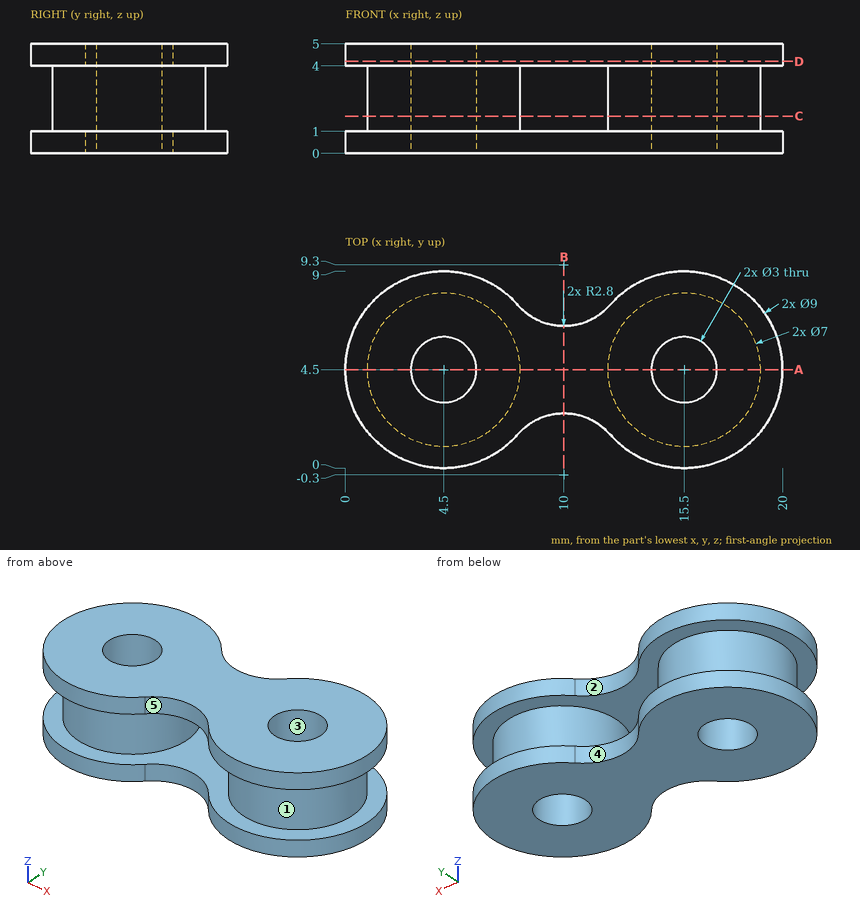
Part print with two shaded views. Sizes in mm from the minimum x, y, z corner. A direction names the side the tool comes from. Give positions to 0.01 mm unless a question says otherwise; leave off trailing zeros. Order: outer loops, then holes, each group sorted by start corner. A loop starts at its lowest first (then second) coordinate and runs counter-clockwise, first axis right, second up. Notation, with made-up numbers: M 55,27.5 L 72,27.5 A19 ccw 72,62.5 Z; hole C 29,87 d2. An arc over 180 degrees is marked long. Use one line per item in the form item = value.
1) Saw through at A-A (y = 4.5). Give the cut face in (x, z), plus the area to 3 significant figures.
Calculated:
outline = M 0,0 L 3,0 L 3,5 L 0,5 L 0,4 L 1,4 L 1,1 L 0,1 Z; M 6,0 L 14,0 L 14,5 L 6,5 Z; M 17,0 L 20,0 L 20,1 L 19,1 L 19,4 L 20,4 L 20,5 L 17,5 Z; hole M 8,1 L 12,1 L 12,4 L 8,4 Z
area = 52.0 mm2
2) Saw through at B-B (x = 10). Give the cut face in (y, z).
Calculated:
outline = M 2.5,0 L 6.5,0 L 6.5,1 L 2.5,1 Z; M 2.5,4 L 6.5,4 L 6.5,5 L 2.5,5 Z
3) Saw through at C-C (z = 1.7). Give the cut face in (x, y), plus the area to 3 significant figures.
Calculated:
outline = C 4.5,4.5 d7; C 15.5,4.5 d7; hole C 4.5,4.5 d3; hole C 15.5,4.5 d3
area = 62.8 mm2
4) Probe probe 1 along X at (y, z) = (4, 3.4); probe 2 along Y at (x, z) = (4.5, 2.75); probe 3 along X at (y, z) = (3.5, 2.85). List the from-to ranges inside material, lowest first.
Calculated:
probe_1 = 1.04 to 3.09, 5.91 to 7.96, 12.04 to 14.09, 16.91 to 18.96
probe_2 = 1 to 3, 6 to 8
probe_3 = 1.15 to 3.38, 5.62 to 7.85, 12.15 to 14.38, 16.62 to 18.85
5) Drop a flat-ended pin along its axis: pin 1 (1 mm diameter, centred on y = 5, z = 3, fed in from +X). Give the stop position or say it passes through.
Calculated:
pin_1 = 19
6) Saw through at D-D (z = 4.2). Give the cut face in (x, y), plus the area to 3 significant figures.
Calculated:
outline = M 7.89,1.54 A2.8 cw 12.11,1.54 A4.5 ccw long 12.11,7.46 A2.8 cw 7.89,7.46 A4.5 ccw long Z; hole C 4.5,4.5 d3; hole C 15.5,4.5 d3
area = 123 mm2
7) Two-plate mould, pull along Y, no slides. Class the marked faces 3, 4 and 5: released by +Y, released by -Y, zero draft, split by the parting line, or undercut.
Calculated:
face_3 = undercut
face_4 = released by +Y
face_5 = released by -Y
8) Tool access for the marked faces 1 and 2: list every direction of +Z, -Z, +X, -X, +Y, -Y with a clear straight run to the whole face (end or side of a thin tool).
Calculated:
face_1 = none
face_2 = +Z, -Z, +Y
